```python
from build123d import *

# Parameters (mm, degrees)
BOSS_EXTRUDE1_DEPTH = 38.1
SKETCH1_3_R         = 77.31506
SKETCH1_3_R_2       = 74.14006
BOSS_EXTRUDE2_DEPTH = 22.225


with BuildPart() as part:
    # Sketch1 → Boss-Extrude1 (new body)
    with BuildSketch(Plane(origin=(0, 0, 0), x_dir=(1, 0, 0), z_dir=(0, 1, 0))):
        with BuildLine():
            Line((13.425619275, -76.140470513), (12.874286311, -73.013705897))
            ThreePointArc((12.874286311, -73.013705897), (-74.14006, 0), (12.874286311, 73.013705897))
            Line((12.874286311, 73.013705897), (13.425619275, 76.140470513))
            ThreePointArc((13.425619275, 76.140470513), (-77.31506, 0), (13.425619275, -76.140470513))
        make_face()
    extrude(amount=BOSS_EXTRUDE1_DEPTH)

    # Sketch1_3 → Boss-Extrude2 (add)
    with BuildSketch(Plane(origin=(0, 0, 0), x_dir=(1, 0, 0), z_dir=(0, 1, 0))):
        Circle(SKETCH1_3_R)
        Circle(SKETCH1_3_R_2, mode=Mode.SUBTRACT)
    extrude(amount=BOSS_EXTRUDE2_DEPTH)


solid = part.part
```
CAD build for the part. Positions are in the model's coordinates, mm. Coordinates: 2 decimals unless noted, no trailing zeros. Write each loop counter-clockwise with the first axis right and the second up, starting at its lowest first coordinate (ties: lowest second). Pieces come first, ordered by that corner, then holes. Notation, with made-up numbers: (-38.5, 33.25) -> (-1.5, 33.25) arc R11 cw to (-1.5, 46.25) -> close; hole circle Ø11 at (65, 41). An arc over 180 degrees is marked (long way). Return JSON: item names as keys, results as strings. Group by question number.
Q1. Cut at D-D, the plane y = 25.5. Give the cut face in (x, z), then the cut area to 3 significant figures.
Q2. Cut at A-A, the plane z = 0. Give the cut face in (x, y) (3 decimals), then the cut area to 3 significant figures.
Q3. Flat gauge pins, fed straight in: pin 1 (1 mm diameter, centred on x = -31.5, y = 7.5, fed in from -Z); pin 2 (10 mm diameter, centred on y = 23, z = 31, fed in from -X); pin 3 (1 mm diameter, centred on x = 48.5, y = 18.5, fed in from -Z). Where does each tip first touch, or does it go through?
Q4. Cut at B-B, the plane x = 0. Give the cut face in (y, z).
Q5. Drill centre lines: line 1 (X direction, y = 20, z = 0); line 2 (Z direction, x = -12, y = 21.5). Where is each one in solid material? Low to high.
Q6. Cut at C-C, the plane y = 7.5. Give the cut face in (x, z).
Returned:
{
 "1": {"outline": "(12.87, -73.01) arc R74.14 cw (long way) to (12.87, 73.01) -> (13.43, 76.14) arc R77.32 ccw (long way) to (13.43, -76.14) -> close", "area": "839 mm2"},
 "2": {"outline": "(-77.315, 0) -> (-74.14, 0) -> (-74.14, 38.1) -> (-77.315, 38.1) -> close; (74.14, 0) -> (77.315, 0) -> (77.315, 22.225) -> (74.14, 22.225) -> close", "area": "192 mm2"},
 "3": {"pin 1": "stops at z = -70.83", "pin 2": "stops at x = -72.81", "pin 3": "stops at z = -60.61"},
 "4": {"outline": "(0, -77.32) -> (38.1, -77.32) -> (38.1, -74.14) -> (0, -74.14) -> close; (0, 74.14) -> (38.1, 74.14) -> (38.1, 77.32) -> (0, 77.32) -> close"},
 "5": {"line 1": "x = -77.32 to -74.14, 74.14 to 77.32", "line 2": "z = -76.38 to -73.16, 73.16 to 76.38"},
 "6": {"outline": "circle Ø154.63 at (0, 0); hole circle Ø148.28 at (0, 0)"}
}
